Part print with two shaded views. Sizes in mm from the minimum x, y, z corner. A direction names the side the tool comes from. Round coordinates to 2 decimals unless told otherwise and drop trailing zeros. Write each loop counter-clockwise with the first axis right and the second up, starting at its lowest first coordinate (ties: lowest second). Pieces come first, ordered by that corner, then holes. Notation, with made-up numbers: M 39.5,71.25 L 81.5,71.25 A19 ccw 81.5,75.25 Z; hole C 7,40 d11. An arc over 180 degrees is marked long. One line per question, with ' | ' between items. Start each with the question number.
1) Tool access for the marked faces 1 and 2: list every direction of +Z, -Z, +X, -X, +Y, -Y with a clear straight run to the whole face (end or side of a thin tool).
2) Saw through at A-A (y = 11). List the corners of the cut face in (x, z) (3 decimals), plus the area to 3 significant figures.
3) Mould opens along X. For the marked faces 3, 4, 5 and 6 say: pulls with the +X half, pulls with the -X half, needs draft (parallel to the pull), parting line crosses it, or undercut.
4) Drop flat-ended pins along their axis: pin 1 Ø5 at (x, z) = (7.5, 3) entering from -Y; pin 2 Ø6 at (x, z) = (6.5, 14.5) entering from -Y (3 decimals); pin 3 Ø2 at (x, z) = (3, 9.5) entering from +Y (3 decimals); pin 4 Ø2 at (x, z) = (4.5, 5.5) entering from -Y. Give the stop position or say it passes through.
5) Saw through at D-D (y = 31.75). List the corners of the cut face in (x, z) (3 decimals), plus the area to 3 significant figures.
6) Saw through at C-C (x = 6.35). List the corners of the cut face in (y, z) (3 decimals).
7) Wall check: probe 1 along Z at (x, y) = (8, 22); probe 2 along Y at (x, z) = (8.5, 1.75); probe 3 along X at (y, z) = (29.5, 13.25). Give the ranges that are in metal, low to high. Write a range as [from, to].
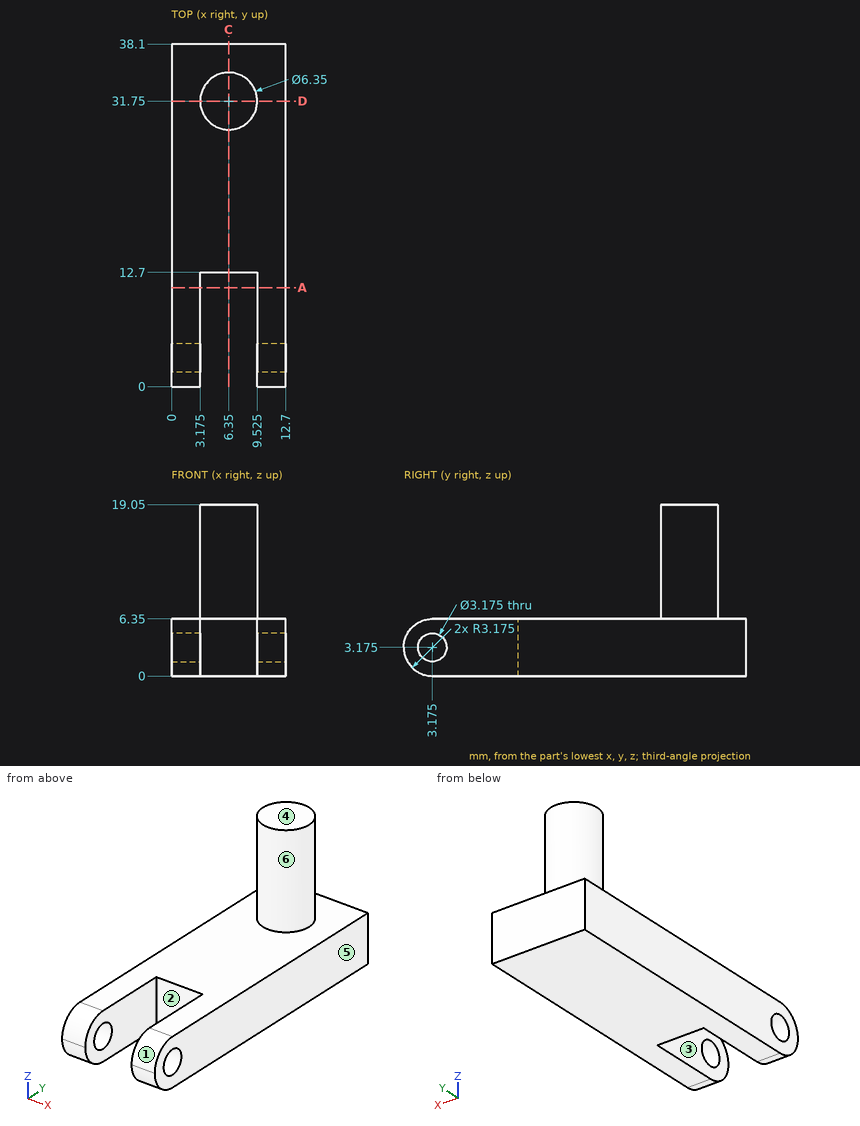
Answer key:
1) face 1: +Z, +X, -X, -Y | face 2: +Z, -Z, -Y
2) outline: M 0,0 L 3.175,0 L 3.175,6.35 L 0,6.35 Z; M 9.525,0 L 12.7,0 L 12.7,6.35 L 9.525,6.35 Z | area: 40.3 mm2
3) face 3: undercut | face 4: needs draft | face 5: pulls with the +X half | face 6: parting line crosses it
4) pin 1: stops at y = 0 | pin 2: stops at y = 28.575 | pin 3: stops at y = 33.885 | pin 4: stops at y = 12.7
5) outline: M 0,0 L 12.7,0 L 12.7,6.35 L 9.525,6.35 L 9.525,19.05 L 3.175,19.05 L 3.175,6.35 L 0,6.35 Z | area: 161 mm2
6) outline: M 12.7,0 L 38.1,0 L 38.1,6.35 L 34.925,6.35 L 34.925,19.05 L 28.575,19.05 L 28.575,6.35 L 12.7,6.35 Z
7) probe 1: z = [0, 6.35] | probe 2: y = [12.7, 38.1] | probe 3: x = [4.11, 8.59]
